```python
from build123d import *

# Parameters (mm, degrees)
SKETCH1_W           = 880
SKETCH1_H           = 410
BOSS_EXTRUDE1_DEPTH = 20
SKETCH3_R           = 30
CUT_EXTRUDE1_DEPTH  = 142
SKETCH4_R           = 4
CUT_EXTRUDE2_DEPTH  = 136
SKETCH5_R           = 6
CUT_EXTRUDE3_DEPTH  = 6
SKETCH7_R           = 20
CUT_EXTRUDE4_DEPTH  = 261


with BuildPart() as part:
    # Sketch1 → Boss-Extrude1 (new body)
    with BuildSketch(Plane(origin=(0, 0, 0), x_dir=(1, 0, 0), z_dir=(0, 1, 0))):
        Rectangle(SKETCH1_W, SKETCH1_H)
    extrude(amount=BOSS_EXTRUDE1_DEPTH)

    # Sketch3 → Cut-Extrude1 (cut)
    with BuildSketch(Plane(origin=(0, 20, 0), x_dir=(1, 0, 0), z_dir=(0, 1, 0))):
        with Locations(Location((-340, 140, 0), (0, 0, 270))):
            Circle(SKETCH3_R)
        with Locations(Location((340, 140, 0), (0, 0, 270))):
            Circle(SKETCH3_R)
        with Locations(Location((340, -140, 0), (0, 0, 270))):
            Circle(SKETCH3_R)
        with Locations(Location((-340, -140, 0), (0, 0, 270))):
            Circle(SKETCH3_R)
    extrude(amount=-CUT_EXTRUDE1_DEPTH, mode=Mode.SUBTRACT)

    # Sketch4 → Cut-Extrude2 (cut)
    with BuildSketch(Plane(origin=(0, 20, 0), x_dir=(1, 0, 0), z_dir=(0, 1, 0))):
        with Locations(Location((-129.655068581, 29.344931419, 0), (0, 0, 270))):
            Circle(SKETCH4_R)
        with Locations(Location((-129.655068581, -29.344931419, 0), (0, 0, 270))):
            Circle(SKETCH4_R)
        with Locations(Location((-188.344931419, -29.344931419, 0), (0, 0, 270))):
            Circle(SKETCH4_R)
        with Locations(Location((-188.344931419, 29.344931419, 0), (0, 0, 270))):
            Circle(SKETCH4_R)
        with Locations(Location((188.344931419, 29.344931419, 0), (0, 0, 270))):
            Circle(SKETCH4_R)
        with Locations(Location((188.344931419, -29.344931419, 0), (0, 0, 270))):
            Circle(SKETCH4_R)
        with Locations(Location((129.655068581, -29.344931419, 0), (0, 0, 270))):
            Circle(SKETCH4_R)
        with Locations(Location((129.655068581, 29.344931419, 0), (0, 0, 270))):
            Circle(SKETCH4_R)
    extrude(amount=-CUT_EXTRUDE2_DEPTH, mode=Mode.SUBTRACT)

    # Sketch5 → Cut-Extrude3 (cut)
    with BuildSketch(Plane.XZ):
        with Locations(Location((-188.344931419, 29.344931419, 0), (0, 0, 270))):
            Circle(SKETCH5_R)
        with Locations(Location((-129.655068581, 29.344931419, 0), (0, 0, 270))):
            Circle(SKETCH5_R)
        with Locations(Location((-129.655068581, -29.344931419, 0), (0, 0, 270))):
            Circle(SKETCH5_R)
        with Locations(Location((-188.344931419, -29.344931419, 0), (0, 0, 270))):
            Circle(SKETCH5_R)
    cut_extrude3 = extrude(amount=-CUT_EXTRUDE3_DEPTH, mode=Mode.SUBTRACT)

    # Mirror1: Cut-Extrude3 across plane
    add(cut_extrude3.mirror(Plane(origin=(0, 0, 0), x_dir=(0, 0, 1), z_dir=(1, 0, 0))), mode=Mode.SUBTRACT)

    # Sketch7 → Cut-Extrude4 (cut)
    with BuildSketch(Plane.XZ):
        with Locations(Location((-250, 0, 0), (0, 0, 270))):
            Circle(SKETCH7_R)
        with Locations(Location((-250, 100, 0), (0, 0, 270))):
            Circle(SKETCH7_R)
        with Locations(Location((-250, -100, 0), (0, 0, 270))):
            Circle(SKETCH7_R)
        with Locations(Location((-70, 100, 0), (0, 0, 270))):
            Circle(SKETCH7_R)
        with Locations(Location((-70, 0, 0), (0, 0, 270))):
            Circle(SKETCH7_R)
        with Locations(Location((-70, -100, 0), (0, 0, 270))):
            Circle(SKETCH7_R)
        with Locations(Location((70, -100, 0), (0, 0, 90))):
            Circle(SKETCH7_R)
        with Locations(Location((70, 0, 0), (0, 0, 90))):
            Circle(SKETCH7_R)
        with Locations(Location((70, 100, 0), (0, 0, 90))):
            Circle(SKETCH7_R)
        with Locations(Location((250, -100, 0), (0, 0, 90))):
            Circle(SKETCH7_R)
        with Locations(Location((250, 100, 0), (0, 0, 90))):
            Circle(SKETCH7_R)
        with Locations(Location((250, 0, 0), (0, 0, 90))):
            Circle(SKETCH7_R)
    extrude(amount=-CUT_EXTRUDE4_DEPTH, mode=Mode.SUBTRACT)


solid = part.part
```
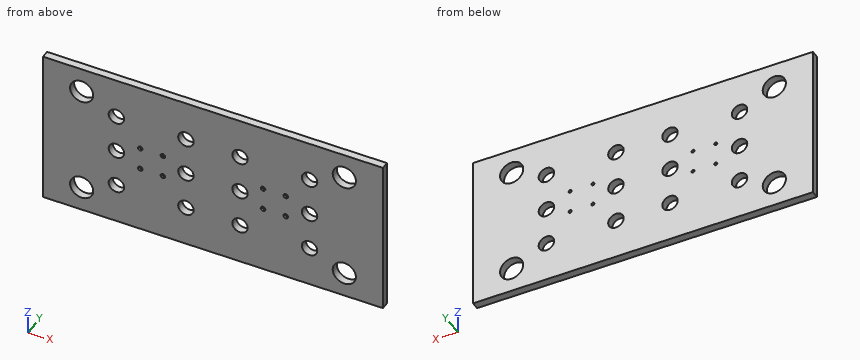
Input: part model. Units: mm. Frame: model coordinates. Coordinates: 2 decimals unless noted, no trailing zeros. Write each loop counter-clockwise with the first axis right and the second up, starting at its lowest first coordinate (ties: lowest second). Pieces come first, ordered by that corner, then holes. Notation, with made-up numbers: M 26.25,43.5 L 53.25,43.5 A32 ccw 53.25,69.5 Z; hole C 84,0.25 d7. An arc over 180 degrees is marked long. Use one line per item in the form item = value.
Q1. Material intervals for probe 1 along Z at (x, y) = (70, 14.5); probe 2 along X at (y, z) = (4.75, -100); probe 3 along Z at (x, y) = (337, 18.75), sorted ascending. Write a range as from..to.
Answer below:
probe_1 = -205..-120, -80..-20, 20..80, 120..205
probe_2 = -440..-270, -230..-90, -50..50, 90..230, 270..440
probe_3 = -205..-169.85, -110.15..110.15, 169.85..205
Q2. Section C-C (z = 100). Return loops of the section in (x, y).
Answer below:
outline = M -440,0 L -270,0 L -270,20 L -440,20 Z; M -230,0 L -90,0 L -90,20 L -230,20 Z; M -50,0 L 50,0 L 50,20 L -50,20 Z; M 90,0 L 230,0 L 230,20 L 90,20 Z; M 270,0 L 440,0 L 440,20 L 270,20 Z
Q3. Section B-B (z = -140). Return loops of the section in (x, y), plus the area to 3 significant figures.
Answer below:
outline = M -440,0 L -370,0 L -370,20 L -440,20 Z; M -310,0 L 310,0 L 310,20 L -310,20 Z; M 370,0 L 440,0 L 440,20 L 370,20 Z
area = 15,200 mm²
Q4. First-contact query: pin 1 (8 mm diameter, centred on x = -245.5, z = 67.5, fed in from -Y). Flat tip, straight axial feed; report the tip coordinate or a pass-through.
Answer below:
pin_1 = 0
Q5. Section A-A (x = -340). Return loops of the section in (y, z), plus the area to 3 significant figures.
Answer below:
outline = M 0,-205 L 20,-205 L 20,-170 L 0,-170 Z; M 0,-110 L 20,-110 L 20,110 L 0,110 Z; M 0,170 L 20,170 L 20,205 L 0,205 Z
area = 5,800 mm²
Q6. Section D-D (x = -70). Return loops of the section in (y, z), plus the area to 3 significant figures.
Answer below:
outline = M 0,-205 L 20,-205 L 20,-120 L 0,-120 Z; M 0,-80 L 20,-80 L 20,-20 L 0,-20 Z; M 0,20 L 20,20 L 20,80 L 0,80 Z; M 0,120 L 20,120 L 20,205 L 0,205 Z
area = 5,800 mm²
